from build123d import *

# Parameters (mm, degrees)
CYLINDER1807_R     = 2.5
CYLINDER1807_DEPTH = 30
CYLINDER1806_R     = 2.5
CYLINDER1806_DEPTH = 30
CYLINDER1808_R     = 2.5
CYLINDER1808_DEPTH = 30
CYLINDER1809_R     = 2.5
CYLINDER1809_DEPTH = 30
BOX716_W           = 100
BOX716_H           = 100
BOX716_DEPTH       = 100
TUBE090_R          = 16
TUBE090_R_2        = 12
TUBE090_DEPTH      = 40
CHAMFER057_SIZE    = 2


with BuildPart() as obj1:
    # Cylinder1807 → Cylinder1807 (new body)
    with BuildSketch(Plane(origin=(58, -19, 26), x_dir=(1, 0, 0), z_dir=(0, 0, 1))):
        Circle(CYLINDER1807_R)
    extrude(amount=CYLINDER1807_DEPTH)


with BuildPart() as compound914:
    # Cylinder1806 → Cylinder1806 (new body)
    with BuildSketch(Plane(origin=(58, 11, 26), x_dir=(1, 0, 0), z_dir=(0, 0, 1))):
        Circle(CYLINDER1806_R)
    extrude(amount=CYLINDER1806_DEPTH)

    # Compound914: union obj1
    add(obj1.part)


with BuildPart() as compound914_1:
    # Compound914 placement: moved
    add(compound914.part.moved(Location((34, 0, 13))))


with BuildPart() as obj2:
    # Cylinder1808 → Cylinder1808 (new body)
    with BuildSketch(Plane(origin=(58, -19, 26), x_dir=(1, 0, 0), z_dir=(0, 0, 1))):
        Circle(CYLINDER1808_R)
    extrude(amount=CYLINDER1808_DEPTH)


with BuildPart() as compound915:
    # Cylinder1809 → Cylinder1809 (new body)
    with BuildSketch(Plane(origin=(58, 11, 26), x_dir=(1, 0, 0), z_dir=(0, 0, 1))):
        Circle(CYLINDER1809_R)
    extrude(amount=CYLINDER1809_DEPTH)

    # Compound916: union obj2
    add(obj2.part)


with BuildPart() as compound915_1:
    # Compound916 placement: moved
    add(compound915.part.moved(Location((0, 0, 13))))

    # Compound915: union Compound914
    add(compound914_1.part)


with BuildPart() as krychle716:
    # Box716 → Box716 (new body)
    with BuildSketch(Plane(origin=(32, -54, -63), x_dir=(1, 0, 0), z_dir=(0, 0, 1))):
        with Locations((50, 50)):
            Rectangle(BOX716_W, BOX716_H)
    extrude(amount=BOX716_DEPTH)


with BuildPart() as cut541:
    # Tube090 → Tube090 (new body)
    with BuildSketch(Plane(origin=(75, 16, 42), x_dir=(1, 0, 0), z_dir=(0, -1, 0))):
        Circle(TUBE090_R)
        Circle(TUBE090_R_2, mode=Mode.SUBTRACT)
    extrude(amount=TUBE090_DEPTH)

    # Chamfer057
    chamfer057_edges = [cut541.edges().sort_by_distance(p)[0] for p in [
        (59, -24, 42),
        (59, 16, 42),
    ]]
    chamfer(chamfer057_edges, length=CHAMFER057_SIZE)

    # Cut533: cut Krychle716
    add(krychle716.part, mode=Mode.SUBTRACT)

    # Cut541: cut Compound915
    add(compound915_1.part, mode=Mode.SUBTRACT)


solid = cut541.part
Can you work these out from the model? Positions are in its coordinate system, mm. A direction names the side the tool comes from. Round coordinates to 2 decimals unless told otherwise and drop trailing zeros. Loops run counter-clockwise (first coordinate to the right, second up) from the corner with the lowest first, then second, coordinate; pieces in that order, holes last. Notation, with made-up numbers: (82, 26) - (138, 26) arc R27 ccw to (138, 52) - close; hole circle Ø1 at (-4.75, 22). An arc over 180 degrees is marked (long way). Write item = value, one per line. Start each with the question number.
(1) If we section it at D-D (y = 12): Please give me the cut outline in (x, z).
(2) If we mould it in two halves opening along Z, with no side actions, what happens to faces 1 (the face through (75, -4, 58)), 2 (the face through (60, -19, 39)), 3 (the face through (75, -4, 54)), 4 (the face through (60.5, -19, 42.7))? For each: released by +Z, released by -Z, zero draft, split by the parting line, or undercut.
(3) If I drill on probe 1 along X at (y, z) = (1.5, 42); probe 2 along X at (y, z) = (-11, 39); probe 3 along Z at (x, y) = (75, -6), over which ranges is the centre line in solid material (lowest first)? Write a range as [from, to].
(4) If we section it at B-B (x = 75): Please give me the cut outline in (y, z).
(5) For faces 5 (the face through (62, -4, 37)), 6 (the face through (90, 11, 39)), 7 (the face through (60.5, 11, 42.7)), which set-ups out of +Z, -Z, +X, -X, +Y, -Y let a thin tool reach every point of the face, with its end or its side?
(6) For P1, Ø1, axis at y = 7.5, z = 54.5, coming from the -X side; P2, Ø1, axis at y = 5, z = 54, coming from the +X side; P3, Ø1, axis at x = 67.5, y = -7, coming from the +Z side, each with a flat end and sliding along its axis, tell me the tip position at first contact or that it passes through.
(7) If we section it at A-A (z = 42): Please give me the cut outline in (x, y).
(8) If we section it at C-C (y = -6): Please give me the cut outline in (x, z), and give its area (3 significant figures).
Ans:
q1.outline = (59.28, 39) arc R16 ccw to (59.8, 37) - (64.09, 37) arc R12 cw (long way) to (85.91, 37) - (90.2, 37) arc R16 ccw to (90.72, 39) - (89.71, 39) - (89.71, 48.3) arc R16 ccw to (60.29, 48.3) - (60.29, 39) - close
q2.face_1 = split by the parting line
q2.face_2 = released by +Z
q2.face_3 = undercut
q2.face_4 = zero draft
q3.probe_1 = [59, 63], [87, 91]
q3.probe_2 = [59.28, 63.38], [86.62, 90.72]
q3.probe_3 = [54, 58]
q4.outline = (-24, 54) - (16, 54) - (16, 56) - (14, 58) - (-22, 58) - (-24, 56) - close
q5.face_5 = -Z, +X, -X, +Y, -Y
q5.face_6 = +Z, +X
q5.face_7 = +Z, -X
q6.P1 = 64.42
q6.P2 = 86.12
q6.P3 = 56.39
q7.outline = (59, -22) - (61, -24) - (63, -24) - (63, 16) - (61, 16) - (59, 14) - (59, 13.29) arc R2.5 cw to (59, 8.71) - (59, -16.71) arc R2.5 cw to (59, -21.29) - close; (87, -24) - (89, -24) - (91, -22) - (91, -21.29) arc R2.5 cw to (91, -16.71) - (91, 8.71) arc R2.5 cw to (91, 13.29) - (91, 14) - (89, 16) - (87, 16) - close
q8.outline = (59.8, 37) - (64.09, 37) arc R12 cw (long way) to (85.91, 37) - (90.2, 37) arc R16 ccw (long way) to start
q8.area = 217 mm²
